Could you check a few things on this model? Use its own coordinates, in mm. Round coordinates to 2 decimals unless told otherwise and drop trailing zeros. Order: outer loops, then holes, each group sorted by start corner. A loop starts at its lowest first (then second) coordinate and runs counter-clockwise, first axis right, second up. Notation, with made-up numbers: M 19,76 L 31,76 A24 cw 31,103 Z; hole C -19,-24 d7. An arc over 180 degrees is marked long. Write each question's results on one line, items separated by ' | '. Start each with the question number.
1. I'm going to push a flat-ended pin straight in: pin 1 (1 mm diameter, centred on y = 84, z = 0.5, fed in from +X). Where does the tip first touch, or does it pass through?
2. Suppose I cut it at C-C on z = 2.05. Give the number of separate pieces and of enclosed holes in the cut face, and give its area (3 significant figures).
3. Suppose I cut it at B-B on x = 42. Write out the boundary of the cut face in (y, z) (3 decimals).
4. Suppose I cut it at A-A on y = 0. Write out the boundary of the cut face in (x, z) (1 decimal).
5. Please list where these lines run through material, in increasing order: L1, parallel to Y at x = 18.5, z = 2.2; L2, parallel to Y at x = -5.5, z = 1; L3, parallel to Y at x = -1.5, z = 2.
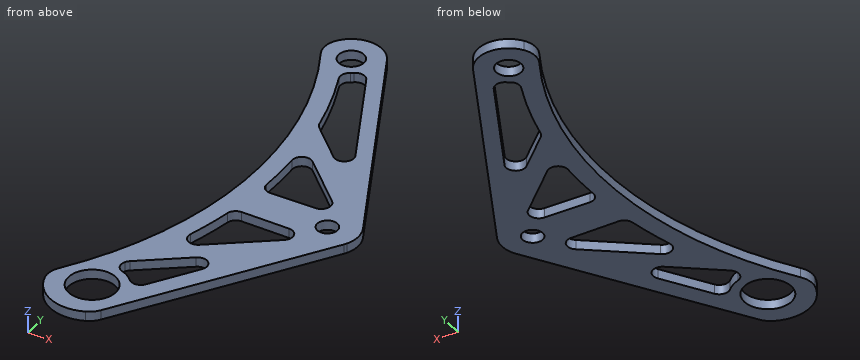
from build123d import *

# Parameters (mm, degrees)
SKETCH1_R           = 7.8105
SKETCH1_R_2         = 3.3655
SKETCH1_R_3         = 4.191
BOSS_EXTRUDE1_DEPTH = 3.175
CUT_EXTRUDE1_DEPTH  = 6.35
FILLET1_R           = 3.175
FILLET5_R           = 7.62


with BuildPart() as part:
    # Sketch1 → Boss-Extrude1 (new body)
    with BuildSketch(Plane.XY):
        with BuildLine():
            Line((8.98309661, 142.414532976), (49.565953559, 65.609056962))
            ThreePointArc((49.565953559, 65.609056962), (50.742856949, 60.862523985), (49.565953559, 56.115991009))
            Line((49.565953559, 56.115991009), (8.177790267, -11.326281223))
            ThreePointArc((8.177790267, -11.326281223), (-6.360706327, -12.437938536), (-13.97, 0))
            ThreePointArc((-13.97, 0), (7.886144716, 68.281846548), (-10.16, 137.668))
            ThreePointArc((-10.16, 137.668), (-2.445131739, 147.529385845), (8.98309661, 142.414532976))
        make_face()
        Circle(SKETCH1_R, mode=Mode.SUBTRACT)
        with Locations((40.582856949, 60.862523985)):
            Circle(SKETCH1_R_2, mode=Mode.SUBTRACT)
        with Locations((0, 137.668)):
            Circle(SKETCH1_R_3, mode=Mode.SUBTRACT)
    extrude(amount=BOSS_EXTRUDE1_DEPTH)

    # Sketch2 → Cut-Extrude1 (cut)
    with BuildSketch(Plane.XY.offset(3.175)):
        with BuildLine():
            ThreePointArc((-0.197260951, 10.983728801), (6.068963009, 9.156904403), (10.192723194, 4.097511946))
            Line((10.192723194, 4.097511946), (31.425957659, 38.69720097))
            Line((31.425957659, 38.69720097), (1.983387122, 15.513785915))
            ThreePointArc((1.983387122, 15.513785915), (0.914134712, 13.238614042), (-0.197260951, 10.983728801))
        make_face()
        with BuildLine():
            Line((6.74876061, 27.348367338), (41.023773829, 54.336902746))
            ThreePointArc((41.023773829, 54.336902746), (40.803440874, 54.325744734), (40.582856949, 54.322023985))
            Line((40.582856949, 54.322023985), (13.144472644, 54.322023985))
            ThreePointArc((13.144472644, 54.322023985), (10.640204067, 40.670739444), (6.74876061, 27.348367338))
        make_face()
        with BuildLine():
            Line((14.194143868, 66.878256842), (40.452496082, 67.401724723))
            Line((40.452496082, 67.401724723), (12.62696706, 92.949274424))
            ThreePointArc((12.62696706, 92.949274424), (14.041969258, 79.951721077), (14.194143868, 66.878256842))
        make_face()
        with BuildLine():
            Line((10.524958055, 103.49970509), (36.307285582, 79.828087082))
            Line((36.307285582, 79.828087082), (6.983478118, 135.325140768))
            ThreePointArc((6.983478118, 135.325140768), (4.680665913, 131.980353508), (0.955265361, 130.364204816))
            ThreePointArc((0.955265361, 130.364204816), (6.450850846, 117.185134994), (10.524958055, 103.49970509))
        make_face()
    extrude(amount=-CUT_EXTRUDE1_DEPTH, mode=Mode.SUBTRACT)

    # Fillet1
    fillet1_edges = [part.edges().sort_by_distance(p)[0] for p in [
        (1.983387122, 15.513785915, 1.5875),
        (-0.197260951, 10.983728801, 1.5875),
        (10.192723194, 4.097511946, 1.5875),
        (31.425957659, 38.69720097, 1.5875),
        (41.023773829, 54.336902746, 1.5875),
        (6.74876061, 27.348367338, 1.5875),
        (13.144472644, 54.322023985, 1.5875),
        (12.62696706, 92.949274424, 1.5875),
        (14.194143868, 66.878256842, 1.5875),
        (40.452496082, 67.401724723, 1.5875),
        (36.307285582, 79.828087082, 1.5875),
        (10.524958055, 103.49970509, 1.5875),
        (0.955265361, 130.364204816, 1.5875),
        (6.983478118, 135.325140768, 1.5875),
    ]]
    fillet(fillet1_edges, radius=FILLET1_R)

    # Fillet5
    # the kernel refuses this fillet: 7.62 mm, written as the material it takes off along each edge
    with BuildSketch(Plane(origin=(49.565953559, 56.115991009, -1.635210381), x_dir=(0.4384758636480836, 0.8987429649227121, 0), z_dir=(0, 0, 1))) as fillet5_piece_1:
        with BuildLine():
            CenterArc((0.408802595, 7.616051271), FILLET5_R, 264.46995043, 7.374672414)
            Line((-0.325519955, 0.031516322), (0, 0))
            ThreePointArc((0, 0), (0.327042076, -0.005264972), (0.654084152, 0))
        make_face()
    extrude(amount=6.445420761, mode=Mode.SUBTRACT)
    with BuildSketch(Plane(origin=(8.177790267, -11.326281223, -6.821790927), x_dir=(-0.8640520418582298, -0.5034024920087542, 0), z_dir=(0, 0, 1))) as fillet5_piece_2:
        with BuildLine():
            CenterArc((1.984520997, -7.583572591), FILLET5_R, 84.39536353, 33.842547752)
            Line((-1.620758554, -0.870424346), (0, 0))
            ThreePointArc((0, 0), (1.364358185, 0.066783583), (2.728716371, 0))
        make_face()
    extrude(amount=16.818581854, mode=Mode.SUBTRACT)
    with BuildSketch(Plane(origin=(-13.97, 0, -10.324988133), x_dir=(0.5491862360699723, 0.8356999928869789, 0), z_dir=(0, 0, 1))) as fillet5_piece_3:
        with BuildLine():
            CenterArc((2.785592727, -7.619579496), FILLET5_R, 90.601931521, 49.710102388)
            ThreePointArc((-3.078254062, -2.753400211), (-1.641438538, -1.262317601), (0, 0))
            ThreePointArc((0, 0), (1.352770433, -0.007105957), (2.705540865, 0))
        make_face()
    extrude(amount=23.824976265, mode=Mode.SUBTRACT)
    with BuildSketch(Plane(origin=(-10.16, 137.668, -14.214457568), x_dir=(0.2798121568434471, 0.96005476764746, 0), z_dir=(0, 0, 1))) as fillet5_piece_4:
        with BuildLine():
            CenterArc((3.553614392, -7.315617329), FILLET5_R, 73.751006034, 62.011444153)
            ThreePointArc((-1.90576169, -1.999640205), (-0.947518647, -1.004930558), (0, 0))
            ThreePointArc((0, 0), (2.842891514, 0.405843561), (5.685783027, 0))
        make_face()
    extrude(amount=31.603915135, mode=Mode.SUBTRACT)


solid = part.part
Filled sheet:
1) pin 1: stops at x = 40.11
2) separate pieces: 1 | enclosed holes: 7 | area: 3,210 mm^2
3) outline: M 43.787,0 L 57.81,0 L 57.81,3.175 L 43.787,3.175 Z; M 63.915,0 L 79.928,0 L 79.928,3.175 L 63.915,3.175 Z
4) outline: M -13.5,0 L -7.8,0 L -7.8,3.2 L -13.5,3.2 Z; M 7.8,0 L 15.1,0 L 15.1,3.2 L 7.8,3.2 Z
5) L1: y = 5.49 to 17.63, 28.24 to 36.6, 54.32 to 66.96, 87.47 to 96.18, 113.53 to 124.4 | L2: y = -12.84 to -5.55, 5.55 to 14.58, 129.11 to 146.21 | L3: y = -13.89 to -7.67, 7.67 to 23.46, 120.23 to 133.75, 141.58 to 147.72
